CAD build for the part. Positions are in the model's coordinates, mm. A direction names the side the tool comes from. Give positions to 0.01 mm unless a question says otherwise; leave off trailing zeros. Order: outer loops, then holes, each group sorted by start corner. A loop starts at its lowest first (then second) coordinate and runs counter-clockwise, first axis right, second up. Notation, with made-up numbers: (-36, -5.5) -> (-15, -5.5) arc R18 ccw to (-15, 24.5) -> close; hole circle Ø4 at (76, 19). An arc over 180 degrees is marked (long way). Use one line per item in the form item = value. Start each with the question number.
1) Probe line 1 (Y direction, x = 0.95, z = -15.25); line 2 (Z direction, x = 1.55, y = -9); line 3 (Y direction, x = 1.65, z = 15). List the from-to ranges inside material, lowest first.
2) Cut at C-C, the plane z = -10. Give the cut face in (x, y), and give its area (3 significant figures).
3) Tool access for faces 1 (the face through (0.986, 3.944, -8.828)), 2 (the face through (0.986, -11.367, 16.71)), 3 (the face through (0.986, -3.944, 8.828)), 4 (the face through (0.986, -5.874, 6.718)), 5 (the face through (0.986, 5.874, -6.718)): list every direction of +Z, -Z, +X, -X, +Y, -Y with a clear straight run to the whole face (end or side of a thin tool).
4) Cut at B-B, the plane y = -9.5. Give the cut face in (x, z), and give its area (3 significant figures).
5) Drop flat-ended pins along their axis: P1, Ø2, axis at y = -2.5, z = -10, coming from the -X side; P2, Ø1, axis at x = 1.5, y = 4.5, coming from the +Z side. Give the stop position or say it passes through.
6) Cut at D-D, the plane y = 6.25. Give the cut face in (x, z), and give its area (3 significant figures).
7) Cut at A-A, the plane x = 1.15. Give the cut face in (y, z), and give its area (3 significant figures).
8) Mould opens along Z. For faces 6 (the face through (0.986, 8.935, -14.696)), 7 (the face through (0.99, -4.06, -9.01)), 8 (the face through (2, 1, 0)) say: pulls with the +Z half, pulls with the -Z half, needs draft (parallel to the pull), parting line crosses it, or undercut.
from build123d import *

# Parameters (mm, degrees)
BOSS_EXTRUDE1_DEPTH  = 2
M2_CLEARANCE_HOLE1_D = 2.4


with BuildPart() as part:
    # Sketch1 → Boss-Extrude1 (new body)
    with BuildSketch(Plane.YZ):
        with BuildLine():
            Line((-10, 13.25), (-1.631578947, 0))
            Line((-1.631578947, 0), (-10, -13.25))
            ThreePointArc((-10, -13.25), (-11.414213562, -16.664213562), (-8, -15.25))
            Line((-8, -15.25), (0, -2.583333333))
            Line((0, -2.583333333), (8, -15.25))
            ThreePointArc((8, -15.25), (11.414213562, -16.664213562), (10, -13.25))
            Line((10, -13.25), (1.631578947, 0))
            Line((1.631578947, 0), (10, 13.25))
            ThreePointArc((10, 13.25), (11.414213562, 16.664213562), (8, 15.25))
            Line((8, 15.25), (0, 2.583333333))
            Line((0, 2.583333333), (-8, 15.25))
            ThreePointArc((-8, 15.25), (-11.414213562, 16.664213562), (-10, 13.25))
        make_face()
    extrude(amount=BOSS_EXTRUDE1_DEPTH)

    # M2 Clearance Hole1 (through all)
    with Locations(Plane(origin=(2, 0, 0), x_dir=(0, 0, -1), z_dir=(1, 0, 0))):
        with Locations((15.25, 10), (15.25, -10), (-15.25, 10), (-15.25, -10)):
            Hole(M2_CLEARANCE_HOLE1_D / 2)


solid = part.part
Result:
q1.line_1 = -12 to -11.2, -8.8 to -8, 8 to 8.8, 11.2 to 12
q1.line_2 = -16.98 to -15.91, -14.59 to -11.67, 11.67 to 14.59, 15.91 to 16.98
q1.line_3 = -11.98 to -11.17, -8.83 to -7.84, 7.84 to 8.83, 11.17 to 11.98
q2.outline = (0, -7.95) -> (2, -7.95) -> (2, -4.68) -> (0, -4.68) -> close; (0, 4.68) -> (2, 4.68) -> (2, 7.95) -> (0, 7.95) -> close
q2.area = 13.1 mm²
q3.face_1 = -Z, +X, -X
q3.face_2 = +X, -X
q3.face_3 = +Z, +X, -X
q3.face_4 = +X, -X, -Y
q3.face_5 = +X, -X, +Y
q4.outline = (0, -17.19) -> (2, -17.19) -> (2, -16.34) -> (0, -16.34) -> close; (0, -14.16) -> (2, -14.16) -> (2, -12.46) -> (0, -12.46) -> close; (0, 12.46) -> (2, 12.46) -> (2, 14.16) -> (0, 14.16) -> close; (0, 16.34) -> (2, 16.34) -> (2, 17.19) -> (0, 17.19) -> close
q4.area = 10.2 mm²
q5.P1 = through
q5.P2 = 10.5
q6.outline = (0, -12.48) -> (2, -12.48) -> (2, -7.31) -> (0, -7.31) -> close; (0, 7.31) -> (2, 7.31) -> (2, 12.48) -> (0, 12.48) -> close
q6.area = 20.7 mm²
q7.outline = (-10, -13.25) arc R2 ccw (long way) to (-8, -15.25) -> (0, -2.58) -> (8, -15.25) arc R2 ccw (long way) to (10, -13.25) -> (1.63, 0) -> (10, 13.25) arc R2 ccw (long way) to (8, 15.25) -> (0, 2.58) -> (-8, 15.25) arc R2 ccw (long way) to (-10, 13.25) -> (-1.63, 0) -> close; hole circle Ø2.4 at (-10, -15.25); hole circle Ø2.4 at (-10, 15.25); hole circle Ø2.4 at (10, -15.25); hole circle Ø2.4 at (10, 15.25)
q7.area = 205 mm²
q8.face_6 = undercut
q8.face_7 = pulls with the -Z half
q8.face_8 = needs draft
